Build history of the part. All positions in model axes, mm. A direction names the side the tool comes from. Give positions to 0.01 mm unless a question says otherwise; leave off trailing zeros. Order: outer loops, then holes, each group sorted by start corner. A loop starts at its lowest first (then second) coordinate and runs counter-clockwise, first axis right, second up. Notation, with made-up numbers: (41, -2) -> (89, -2) arc R16 ccw to (89, 17) -> close; hole circle Ø6 at (-14, 77.25). An arc over 180 degrees is marked (long way). One line per item, written item: value. Start each with the question number.
(1) Saw through at B-B on y = 3. Give the cut face in (x, z), plus the area to 3 significant figures.
(2) Saw through at D-D on y = 16. Give the cut face in (x, z), plus the area to 3 significant figures.
(3) Probe line 1 (Z direction, x = 0, y = 25.1); line 2 (Z direction, x = 3, y = -16.5); line 3 (Z direction, x = 4, y = -12.5). List the from-to ranges inside material, lowest first.
(4) Which spindle directions (+Z, -Z, +X, -X, +Y, -Y) get a long thin tool onto all of the face, cutting with end or side? Do faces 1 (the cylindrical face through (-11, -10.2, 33.9)), 2 (the flat face through (7, 7, 44)), 3 (the flat face through (0, 0, -30)), 4 (the flat face through (17.717, 17.638, 37.098)), 5 (the flat face through (-3.575, -3.496, 40.958)). Say none if no direction does.
(5) Saw through at A-A on z = 0. Give the cut face in (x, y).
(6) Saw through at C-C on x = -5.5. Give the cut face in (y, z), plus the area to 3 significant figures.
(7) Pin check, flat tip, straight feed: pin 1 (6 mm diameter, centred on y = -6.5, z = 34, fed in from +X). Stop position of the tip, or through.
(8) Two-plate mould, pull along X, no slides. Class faces 6 (the flat face through (-25, 0, 0)), 7 (the flat face through (-6, 27.5, 0)), 8 (the cylindrical face through (0.867, 24.542, -3.905)), 9 (the flat face through (0, 21.5, 0)): +X half, -X half, draft (parallel to the pull), parting line (faces both ways), or undercut.
```python
from build123d import *

# Parameters (mm, degrees)
SKETCH_1_W                  = 50
SKETCH_1_H                  = 55
EXTRUDE_1_DEPTH             = 30
SKETCH_2_R                  = 15
EXTRUDE_2_DEPTH             = 8
EXTRUDE_3_DEPTH             = 6
EXTRUDE_3_DIRECTION_2_REACH = 79.494
SKETCH_4_R                  = 4
CUT_EXTRUDE_1_DEPTH         = 6


with BuildPart() as part:
    # 草图1 → 凸台-拉伸1 (new, symmetric)
    with BuildSketch(Plane.XY):
        Rectangle(SKETCH_1_W, SKETCH_1_H)
    extrude(amount=EXTRUDE_1_DEPTH, both=True)

    # 草图2 → 凸台-拉伸2 (add)
    with BuildSketch(Plane.XY.offset(30)):
        Circle(SKETCH_2_R)
    extrude(amount=EXTRUDE_2_DEPTH)

    # 草图3 → 凸台-拉伸3 (add)
    with BuildSketch(Plane.XY.offset(38)):
        Polygon((14.849242405, 20.506096654), (-6.363961031, -0.707106781), (-0.707106781, -6.363961031), (20.506096654, 14.849242405), align=None)
    extrude(amount=EXTRUDE_3_DEPTH)

    # 草图3 → 凸台-拉伸3 direction 2 (add, up to next)
    with BuildSketch(Plane.XY.offset(38), mode=Mode.PRIVATE) as extrude_3_direction_2_sk1:
        Polygon((14.849242405, 20.506096654), (-6.363961031, -0.707106781), (-0.707106781, -6.363961031), (20.506096654, 14.849242405), align=None)
    extrude_3_direction_2_tool1 = extrude(extrude_3_direction_2_sk1.sketch, amount=-EXTRUDE_3_DIRECTION_2_REACH, mode=Mode.PRIVATE) - part.part
    add(extrude_3_direction_2_tool1.solids().sort_by_distance((7.071068, 7.071068, 38))[0])

    # 草图4 → 切除-拉伸1 (cut)
    with BuildSketch(Plane(origin=(0, 27.5, 0), x_dir=(1, 0, 0), z_dir=(0, 1, 0))):
        with Locations(Location((0, 0, 0), (0, 0, 180))):
            Circle(SKETCH_4_R)
    extrude(amount=-CUT_EXTRUDE_1_DEPTH, mode=Mode.SUBTRACT)


solid = part.part
```
Results below:
1. outline: (-25, -30) -> (25, -30) -> (25, 30) -> (14.7, 30) -> (14.7, 38) -> (8.66, 38) -> (8.66, 44) -> (-2.66, 44) -> (-2.66, 38) -> (-14.7, 38) -> (-14.7, 30) -> (-25, 30) -> close
1. area: 3,300 mm²
2. outline: (-25, -30) -> (25, -30) -> (25, 30) -> (19.36, 30) -> (19.36, 44) -> (10.34, 44) -> (10.34, 30) -> (-25, 30) -> close
2. area: 3,130 mm²
3. line 1: z = -30 to -4, 4 to 30
3. line 2: z = -30 to 30
3. line 3: z = -30 to 38
4. face 1: +Z
4. face 2: +Z, +X, -X, +Y, -Y
4. face 3: -Z, +X, -X, +Y, -Y
4. face 4: +Z, +X, +Y
4. face 5: +Z, -X, -Y
5. outline: (-25, -27.5) -> (25, -27.5) -> (25, 27.5) -> (4, 27.5) -> (4, 21.5) -> (-4, 21.5) -> (-4, 27.5) -> (-25, 27.5) -> close
6. outline: (-27.5, -30) -> (27.5, -30) -> (27.5, 30) -> (13.96, 30) -> (13.96, 38) -> (0.16, 38) -> (0.16, 44) -> (-1.57, 44) -> (-1.57, 38) -> (-13.96, 38) -> (-13.96, 30) -> (-27.5, 30) -> close
6. area: 3,530 mm²
7. pin 1: stops at x = 14.59
8. face 6: -X half
8. face 7: draft
8. face 8: undercut
8. face 9: undercut
